```python
from build123d import *

# Parameters (mm, degrees)
SKETCH1_W           = 200
SKETCH1_H           = 200
BOSS_EXTRUDE1_DEPTH = 2
SKETCH2_R           = 2
CUT_EXTRUDE1_DEPTH  = 13
SKETCH3_R           = 2
CUT_EXTRUDE2_DEPTH  = 142.435497666
SKETCH4_R           = 2
CUT_EXTRUDE3_DEPTH  = 13
SKETCH5_W           = 2
SKETCH5_H           = 50
BOSS_EXTRUDE2_DEPTH = 16.5
SKETCH6_R           = 2
SKETCH6_W           = 13
SKETCH6_H           = 15
CUT_EXTRUDE4_DEPTH  = 154.545595834
SKETCH7_R           = 2
CUT_EXTRUDE5_DEPTH  = 154.545595834
CUT_EXTRUDE6_DEPTH  = 10
SKETCH11_W          = 216.5
SKETCH11_H          = 2
BOSS_EXTRUDE3_DEPTH = 50
CUT_EXTRUDE8_DEPTH  = 10
CUT_EXTRUDE9_DEPTH  = 10
CUT_EXTRUDE10_DEPTH = 10
SKETCH17_R          = 2
CUT_EXTRUDE11_DEPTH = 10
SKETCH18_R          = 2
CUT_EXTRUDE12_DEPTH = 10
CUT_EXTRUDE13_DEPTH = 10
CUT_EXTRUDE14_DEPTH = 10
CUT_EXTRUDE15_DEPTH = 10
SKETCH22_R          = 2
CUT_EXTRUDE16_DEPTH = 10
SKETCH23_W          = 13
SKETCH23_H          = 26
CUT_EXTRUDE17_DEPTH = 10
CUT_EXTRUDE20_DEPTH = 10


with BuildPart() as part:
    # Sketch1 → Boss-Extrude1 (new body)
    with BuildSketch(Plane.XY):
        Rectangle(SKETCH1_W, SKETCH1_H)
    extrude(amount=BOSS_EXTRUDE1_DEPTH)

    # Sketch2 → Cut-Extrude1 (cut)
    with BuildSketch(Plane.XY.offset(2)):
        with Locations((90.5, 70)):
            Circle(SKETCH2_R)
        with Locations((90.5, -70)):
            Circle(SKETCH2_R)
    extrude(amount=-CUT_EXTRUDE1_DEPTH, mode=Mode.SUBTRACT)

    # Sketch3 → Cut-Extrude2 (cut, through all)
    with BuildSketch(Plane.XY.offset(2)):
        with Locations((-90.5, -40)):
            Circle(SKETCH3_R)
        with Locations((-90.5, -80)):
            Circle(SKETCH3_R)
    extrude(amount=-CUT_EXTRUDE2_DEPTH, mode=Mode.SUBTRACT)

    # Sketch4 → Cut-Extrude3 (cut)
    with BuildSketch(Plane.XY.offset(2)):
        with Locations((-50, -45)):
            Circle(SKETCH4_R)
        with Locations((-50, -80)):
            Circle(SKETCH4_R)
        with Locations((26.5, -45)):
            Circle(SKETCH4_R)
        with Locations((26.5, -80)):
            Circle(SKETCH4_R)
    extrude(amount=-CUT_EXTRUDE3_DEPTH, mode=Mode.SUBTRACT)

    # Sketch5 → Boss-Extrude2 (add)
    with BuildSketch(Plane.ZY.offset(100)):
        with Locations((1, 75)):
            Rectangle(SKETCH5_W, SKETCH5_H)
    extrude(amount=BOSS_EXTRUDE2_DEPTH)

    # Sketch6 → Cut-Extrude4 (cut, through all)
    with BuildSketch(Plane.XY.offset(2)):
        with Locations((-111.5, 70)):
            Circle(SKETCH6_R)
        with Locations((-88.5, 70)):
            Circle(SKETCH6_R)
        with Locations((-100, 66)):
            Rectangle(SKETCH6_W, SKETCH6_H)
    extrude(amount=-CUT_EXTRUDE4_DEPTH, mode=Mode.SUBTRACT)

    # Sketch7 → Cut-Extrude5 (cut, through all)
    with BuildSketch(Plane.XY.offset(2)):
        with Locations((75, 85)):
            Circle(SKETCH7_R)
        with Locations((78, -35)):
            Circle(SKETCH7_R)
        with Locations((-78, -35)):
            Circle(SKETCH7_R)
        with Locations((-75, 85)):
            Circle(SKETCH7_R)
    extrude(amount=-CUT_EXTRUDE5_DEPTH, mode=Mode.SUBTRACT)

    # Sketch8 → Cut-Extrude6 (cut)
    with BuildSketch(Plane.XY.offset(2)):
        with BuildLine():
            Line((67, 95), (67, 32))
            ThreePointArc((67, 32), (65, 30), (63, 32))
            Line((63, 32), (63, 95))
            ThreePointArc((63, 95), (65, 97), (67, 95))
        make_face()
    extrude(amount=-CUT_EXTRUDE6_DEPTH, mode=Mode.SUBTRACT)

    # Sketch11 → Boss-Extrude3 (add)
    with BuildSketch(Plane(origin=(0, 100, 0), x_dir=(1, 0, 0), z_dir=(0, 1, 0))):
        with Locations((-8.25, -1)):
            Rectangle(SKETCH11_W, SKETCH11_H)
    extrude(amount=BOSS_EXTRUDE3_DEPTH)

    # Sketch12 → Cut-Extrude8 (cut)
    with BuildSketch(Plane.XY.offset(2)):
        with BuildLine():
            Line((63, 90.479574642), (63, 140))
            ThreePointArc((63, 140), (65, 142), (67, 140))
            Line((67, 140), (67, 90.479574642))
            ThreePointArc((67, 90.479574642), (65, 88.479574642), (63, 90.479574642))
        make_face()
    extrude(amount=-CUT_EXTRUDE8_DEPTH, mode=Mode.SUBTRACT)

    # Sketch15 → Cut-Extrude9 (cut)
    with BuildSketch(Plane.XY.offset(2)):
        with BuildLine():
            Line((-78, -33), (78, -33))
            ThreePointArc((78, -33), (80, -35), (78, -37))
            Line((78, -37), (-78, -37))
            ThreePointArc((-78, -37), (-80, -35), (-78, -33))
        make_face()
    extrude(amount=-CUT_EXTRUDE9_DEPTH, mode=Mode.SUBTRACT)

    # Sketch16 → Cut-Extrude10 (cut)
    with BuildSketch(Plane.XY.offset(2)):
        with BuildLine():
            Line((-75, 87), (75, 87))
            ThreePointArc((75, 87), (77, 85), (75, 83))
            Line((75, 83), (-75, 83))
            ThreePointArc((-75, 83), (-77, 85), (-75, 87))
        make_face()
    extrude(amount=-CUT_EXTRUDE10_DEPTH, mode=Mode.SUBTRACT)

    # Sketch17 → Cut-Extrude11 (cut)
    with BuildSketch(Plane.XY.offset(2)):
        with Locations((90.5, 120)):
            Circle(SKETCH17_R)
    extrude(amount=-CUT_EXTRUDE11_DEPTH, mode=Mode.SUBTRACT)

    # Sketch18 → Cut-Extrude12 (cut)
    with BuildSketch(Plane.XY.offset(2)):
        with Locations((-90.5, 120)):
            Circle(SKETCH18_R)
    extrude(amount=-CUT_EXTRUDE12_DEPTH, mode=Mode.SUBTRACT)

    # Sketch19 → Cut-Extrude13 (cut)
    with BuildSketch(Plane.XY.offset(2)):
        with BuildLine():
            Line((15, 4), (50, 4))
            ThreePointArc((50, 4), (52, 2), (50, 0))
            Line((50, 0), (15, 0))
            ThreePointArc((15, 0), (13, 2), (15, 4))
        make_face()
    extrude(amount=-CUT_EXTRUDE13_DEPTH, mode=Mode.SUBTRACT)

    # Sketch20 → Cut-Extrude14 (cut)
    with BuildSketch(Plane.XY.offset(2)):
        with BuildLine():
            Line((-58, -43), (-33, -43))
            ThreePointArc((-33, -43), (-31, -45), (-33, -47))
            Line((-33, -47), (-58, -47))
            ThreePointArc((-58, -47), (-60, -45), (-58, -43))
        make_face()
        with BuildLine():
            Line((-58, -78), (-33, -78))
            ThreePointArc((-33, -78), (-31, -80), (-33, -82))
            Line((-33, -82), (-58, -82))
            ThreePointArc((-58, -82), (-60, -80), (-58, -78))
        make_face()
        with BuildLine():
            Line((12, -43), (37, -43))
            ThreePointArc((37, -43), (39, -45), (37, -47))
            Line((37, -47), (12, -47))
            ThreePointArc((12, -47), (10, -45), (12, -43))
        make_face()
        with BuildLine():
            Line((12, -78), (37, -78))
            ThreePointArc((37, -78), (39, -80), (37, -82))
            Line((37, -82), (12, -82))
            ThreePointArc((12, -82), (10, -80), (12, -78))
        make_face()
    extrude(amount=-CUT_EXTRUDE14_DEPTH, mode=Mode.SUBTRACT)

    # Sketch21 → Cut-Extrude15 (cut)
    with BuildSketch(Plane.XY.offset(2)):
        with BuildLine():
            Line((-88.5, 140), (-88.5, 100))
            ThreePointArc((-88.5, 100), (-90.5, 98), (-92.5, 100))
            Line((-92.5, 100), (-92.5, 140))
            ThreePointArc((-92.5, 140), (-90.5, 142), (-88.5, 140))
        make_face()
    extrude(amount=-CUT_EXTRUDE15_DEPTH, mode=Mode.SUBTRACT)

    # Sketch22 → Cut-Extrude16 (cut)
    with BuildSketch(Plane.XY.offset(2)):
        with Locations((-100, 53.5)):
            Circle(SKETCH22_R)
        with Locations((-100, 104.5)):
            Circle(SKETCH22_R)
    extrude(amount=-CUT_EXTRUDE16_DEPTH, mode=Mode.SUBTRACT)

    # Sketch23 → Cut-Extrude17 (cut)
    with BuildSketch(Plane.XY.offset(2)):
        with Locations((-100, 86.5)):
            Rectangle(SKETCH23_W, SKETCH23_H)
    extrude(amount=-CUT_EXTRUDE17_DEPTH, mode=Mode.SUBTRACT)

    # Sketch24 → Cut-Extrude20 (cut)
    with BuildSketch(Plane.XY.offset(2)):
        with BuildLine():
            Line((-90.5, 75), (-90.5, 85))
            ThreePointArc((-90.5, 85), (-88.5, 87), (-86.5, 85))
            Line((-86.5, 85), (-86.5, 75))
            ThreePointArc((-86.5, 75), (-88.5, 73), (-90.5, 75))
        make_face()
        with BuildLine():
            Line((-113.741584086, 75), (-113.741584086, 85))
            ThreePointArc((-113.741584086, 85), (-111.741584086, 87), (-109.741584086, 85))
            Line((-109.741584086, 85), (-109.741584086, 75))
            ThreePointArc((-109.741584086, 75), (-111.741584086, 73), (-113.741584086, 75))
        make_face()
    extrude(amount=-CUT_EXTRUDE20_DEPTH, mode=Mode.SUBTRACT)


solid = part.part
```
The listing builds one solid part. Answer for the finished solid, in the listing's coordinates (mm). Give positions to 0.01 mm unless a question says otherwise; leave off trailing zeros. Write each loop counter-clockwise with the first axis right and the second up, starting at its lowest first coordinate (ties: lowest second). Pieces come first, ordered by that corner, then holes. Notation, with made-up numbers: (56.5, 11) -> (76.5, 11) arc R10 cw to (76.5, 27) -> close; hole circle Ø3 at (-32, -37.5). An arc over 180 degrees is marked (long way). Write item = value, one per line. Start each with the question number.
1) The part is cut by section D-D, the plane y = 94. Determine the outline of the cut face in (x, z).
2) The part is cut by section B-B, the plane y = 38.5. Determine the outline of the cut face in (x, z), and give its area (3 significant figures).
3) The part is cut by section C-C, the plane x = -38.5. Determine the outline of the cut face in (y, z).
4) Straight lines are drawn through the part: line 1 along X through (y, z) = (87.5, 0.15); line 2 along Y through (x, z) = (-19, 0.6); line 3 along Y through (x, z) = (-56, 1.8). For each, find the intervals that lie inside material, in ascending order.
5) This flat-tipped pin is pushed along its axis until it touches: pin 1 (5 mm diameter, centred on x = 90.5, y = 70, fed in from +Z). Where does it stop, or does it pass through?
6) The part is cut by section A-A, the plane x = 70. Determine the outline of the cut face in (y, z), and give its area (3 significant figures).
Solutions:
q1.outline = (-116.5, 0) -> (-106.5, 0) -> (-106.5, 2) -> (-116.5, 2) -> close; (-93.5, 0) -> (63, 0) -> (63, 2) -> (-93.5, 2) -> close; (67, 0) -> (100, 0) -> (100, 2) -> (67, 2) -> close
q2.outline = (-100, 0) -> (63, 0) -> (63, 2) -> (-100, 2) -> close; (67, 0) -> (100, 0) -> (100, 2) -> (67, 2) -> close
q2.area = 392 mm²
q3.outline = (-100, 0) -> (-82, 0) -> (-82, 2) -> (-100, 2) -> close; (-78, 0) -> (-47, 0) -> (-47, 2) -> (-78, 2) -> close; (-43, 0) -> (-37, 0) -> (-37, 2) -> (-43, 2) -> close; (-33, 0) -> (83, 0) -> (83, 2) -> (-33, 2) -> close; (87, 0) -> (150, 0) -> (150, 2) -> (87, 2) -> close
q4.line_1 = -116.5 to -106.5, -93.5 to 63, 67 to 100
q4.line_2 = -100 to -37, -33 to 83, 87 to 150
q4.line_3 = -100 to -82, -78 to -47, -43 to -37, -33 to 83, 87 to 150
q5.pin_1 = 2
q6.outline = (-100, 0) -> (-37, 0) -> (-37, 2) -> (-100, 2) -> close; (-33, 0) -> (83, 0) -> (83, 2) -> (-33, 2) -> close; (87, 0) -> (150, 0) -> (150, 2) -> (87, 2) -> close
q6.area = 484 mm²
